Geometry check sheet. Reference: the model listing, model coordinates, mm. Face numbers are marked on the shaded views. A direction names the side the tool comes from. Give positions to 0.01 mm unless a question says otherwise; leave off trailing zeros. Write each loop counter-clockwise with the first axis right and the second up, starting at its lowest first coordinate (ties: lowest second). Pieces come first, ordered by that corner, then holes. Notation, with made-up numbers: M -18,-33 L 4,-33 A14 cw 4,-21 Z; hole C 38.25,46 d6. An arc over 180 degrees is marked long. Use one line per item in the form item = value. Start each with the question number.
Autodesk Inventor part; units mm, degrees
ref_plane "YZ Plane" through (0, 0, 0) normal (1, 0, 0) x (0, 1, 0)
ref_plane "XZ Plane" through (0, 0, 0) normal (0, 1, 0) x (-1, 0, 0)
ref_plane "XY Plane" through (0, 0, 0) normal (0, 0, 1) x (1, 0, 0)
sketch "Sketch3" plane through (0, 0, 0) normal (0, 0, 1) x (1, 0, 0)
  line L0 (-10.1, 25) -> (10.1, 25)
  line L1 (10.1, 25) -> (10.1, -25)
  line L2 (10.1, -25) -> (-10.1, -25)
  line L3 (-10.1, -25) -> (-10.1, 25)
  point P0 (0, 0)
  dimension "d26" = 20.2
  dimension "d27" = 50
extrude "Extrusion3" add sketch "Sketch3" along normal blind 1.8
sketch "Sketch4" plane through (0, 0, 1.8) normal (0, 0, 1) x (1, 0, 0)
  line L0 (-8.1, 23) -> (8.1, 23)
  line L1 (8.1, -23) -> (-8.1, -23)
  line L2 (-8.1, 0) -> (-8.1, 2.5)
  line L3 (-8.1, 2.5) -> (8.1, 2.5)
  line L4 (8.1, 4.5) -> (-8.1, 4.5)
  line L5 (-8.1, 0) -> (-8.1, -2.5)
  line L6 (-8.1, -2.5) -> (8.1, -2.5)
  line L7 (8.1, -4.5) -> (-8.1, -4.5)
  line L8 (-8.1, 4.5) -> (-8.1, 23)
  line L9 (8.1, 23) -> (8.1, 4.5)
  line L10 (8.1, 2.5) -> (8.1, -2.5)
  line L11 (8.1, -4.5) -> (8.1, -23)
  line L12 (-10.1, 25) -> (-10.1, -25)
  line L13 (10.1, -25) -> (10.1, 25)
  line L14 (-10.1, 25) -> (10.1, 25)
  line L15 (10.1, 25) -> (10.1, -25)
  line L16 (10.1, -25) -> (-10.1, -25)
  line L17 (-10.1, -25) -> (-10.1, 25)
  line L18 (-8.1, -23) -> (-8.1, -4.5)
  line L19 (-8.1, -2.5) -> (-8.1, 2.5)
  point P0 (0, 0)
  dimension "d39" = 2.5
  dimension "d40" = 2.5
  dimension "d44" = 2
  dimension "d45" = 2
  dimension "d48" = 2
  dimension "d49" = 2
  dimension "d50" = 2
  dimension "d51" = 2
  dimension "d52" = 2
  dimension "d53" = 2
  dimension "d56" = 2
  dimension "d57" = 2
extrude "Extrusion4" add sketch "Sketch4" along normal blind 8.2
sketch "Sketch5" plane through (10.1, -25, 0) normal (1, 0, 0) x (0, 0, -1)
  line L0 (-1.8, 27.5) -> (-10, 27.5)
  line L1 (-1.8, 22.5) -> (-10, 22.5)
  line L2 (-10, 27.5) -> (-1.8, 27.5)
  line L3 (-1.8, 27.5) -> (-1.8, 22.5)
  line L4 (-1.8, 22.5) -> (-10, 22.5)
  line L5 (-10, 22.5) -> (-10, 27.5)
  point P0 (0, 25)
extrude "Extrusion5" cut sketch "Sketch5" against normal blind 8.2
sketch "Sketch6" plane through (-10.1, -25, 0) normal (-1, 0, 0) x (0, 0, 1)
  line L0 (1.8, 27.5) -> (1.8, 22.5)
  line L1 (1.8, 22.5) -> (6.8, 22.5)
  line L2 (6.8, 22.5) -> (6.8, 27.5)
  line L3 (6.8, 27.5) -> (1.8, 27.5)
  line L4 (1.8, 27.5) -> (1.8, 22.5)
  point P0 (0, 25)
  dimension "d60" = 5
  dimension "d61" = 5
extrude "Extrusion6" cut sketch "Sketch6" against normal blind 8.2
sketch "Sketch7" plane through (-10.1, -25, 0) normal (-1, 0, 0) x (0, 0, 1)
  line L0 (0, 50) -> (10, 50)
  line L1 (0, 0) -> (0, 50)
  line L2 (0, 0) -> (10, 0)
  line L3 (10, 50) -> (10, 0)
  line L4 (10, 29.5) -> (10, 48)
  line L5 (10, 20.5) -> (10, 2)
  point P0 (0, 25)
  point P1 (4.5, 40)
  point P2 (4.5, 10)
  dimension "d66" = 10
  dimension "d67" = 4.5
hole "Hole1" at (-10.1, 15, 4.5) at (-10.1, -15, 4.5) direction (1, 0, 0) diameter 2.6 depth 2 tip angle 118
chamfer "Chamfer3" distance 1 angle 45 2 edges at (-8.1, -15, 3.2) (-8.1, 15, 3.2)
sketch "Sketch10" plane through (10.1, -25, 0) normal (1, 0, 0) x (0, 0, -1)
  circle A0 centre (-4.5, 40) radius 2.3
  circle A1 centre (-4.5, 10) radius 2.3
  point P0 (0, 25)
hole "Hole6" at (10.1, -15, 4.5) at (10.1, 15, 4.5) direction (-1, 0, 0) diameter 2.6 depth 2 tip angle 118
sketch "Sketch11" plane through (-10.1, 2.5, 1.8) normal (0, -1, 0) x (1, 0, 0)
  line L0 (2, 8.2) -> (20.2, 8.2)
  line L1 (20.2, 8.2) -> (18.2, 8.2)
  line L2 (18.2, 8.2) -> (18.2, 5)
  line L3 (18.2, 5) -> (20.2, 5)
  line L4 (20.2, 5) -> (20.2, 8.2)
  point P0 (10.1, -1.8)
  dimension "d141" = 2
  dimension "d142" = 3.2
extrude "Extrusion9" add sketch "Sketch11" along normal blind 10
chamfer "Chamfer4" distance 1 angle 45 2 edges at (8.1, 15, 5.8) (8.1, -15, 5.8)
properties part number "digit_holder_C"
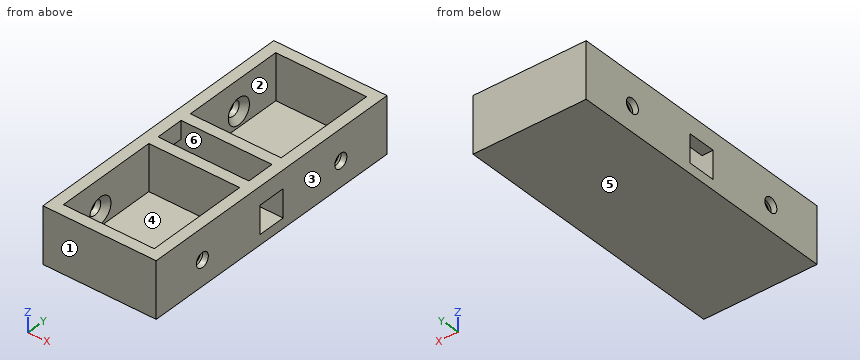
(1) Sectioned sample at B-B, the plane x = -4.75. Record the boundary of the cut face in (y, z).
(2) Sectioned sample at C-C, the plane z = 8.25. Record the boundary of the cut face in (x, y), plus the area to 3 significant figures.
(3) Tool access check on the marked faces 4, 5 and 6. Record the directions out of +Z, -Z, +X, -X, +Y, -Y that give a thin tool (end or side, any length) a straight path to the whole face; none if there is none.
(4) Sectioned sample at D-D, the plane y = 0. Record the boundary of the cut face in (x, z).
(5) Sectioned sample at A-A, the plane y = -15. Record the boundary of the cut face in (x, z), plus the area to 3 significant figures.
(6) Thickness scan on probe 1 along Y at (x, z) = (-9.35, 4.5); probe 2 along Y at (x, z) = (5, 5.5); probe 3 along X at (y, z) = (21, 3). Record the ranges inside material, lowest first. Write a range as [from, to].
(7) Depth check by flat-ended pin: pin 1 (1 mm diameter, centred on x = -6.5, y = -11.5, fed in from +Z). Enter the tip coordinate at first touch or a pass-through.
(8) Draft check along X on the marked faces 1, 2 and 3. Enter one of: released by +X, released by -X, zero draft, split by the parting line, or undercut.
Numbers:
q1.outline = M -25,0 L 25,0 L 25,10 L 23,10 L 23,1.8 L 4.5,1.8 L 4.5,10 L 2.5,10 L 2.5,1.8 L -2.5,1.8 L -2.5,10 L -4.5,10 L -4.5,1.8 L -23,1.8 L -23,10 L -25,10 Z
q2.outline = M -10.1,-25 L 10.1,-25 L 10.1,25 L -10.1,25 Z; hole M -8.1,-23 L 8.1,-23 L 8.1,-4.5 L -8.1,-4.5 Z; hole M -8.1,-2.5 L 8.1,-2.5 L 8.1,2.5 L -8.1,2.5 Z; hole M -8.1,4.5 L 8.1,4.5 L 8.1,23 L -8.1,23 Z
q2.area = 330 mm2
q3.face_4 = +Z
q3.face_5 = -Z, +X, -X, +Y, -Y
q3.face_6 = none
q4.outline = M -10.1,0 L 10.1,0 L 10.1,1.8 L -10.1,1.8 Z; M -10.1,6.8 L -8.1,6.8 L -8.1,10 L -10.1,10 Z; M 8.1,6.8 L 10.1,6.8 L 10.1,10 L 8.1,10 Z
q5.outline = M -10.1,0 L 10.1,0 L 10.1,3.2 L 9.1,3.2 L 8.1,2.2 L 8.1,1.8 L -8.1,1.8 L -8.1,2.2 L -9.1,3.2 L -10.1,3.2 Z; M -10.1,5.8 L -9.1,5.8 L -8.1,6.8 L -8.1,10 L -10.1,10 Z; M 8.1,6.8 L 9.1,5.8 L 10.1,5.8 L 10.1,10 L 8.1,10 Z
q5.area = 56.8 mm2
q6.probe_1 = [-25, -16.3], [-13.7, -2.5], [2.5, 13.7], [16.3, 25]
q6.probe_2 = [-25, -23], [-4.5, -2.5], [2.5, 4.5], [23, 25]
q6.probe_3 = [-10.1, -8.1], [8.1, 10.1]
q7.pin_1 = 1.8
q8.face_1 = zero draft
q8.face_2 = undercut
q8.face_3 = released by +X
